Source: CAD feature listing. Evaluate the final solid. Frame: model axes, mm. A direction names the side the tool comes from. Coordinates: 2 decimals unless noted, no trailing zeros. Write each loop counter-clockwise with the first axis right and the second up, starting at its lowest first coordinate (ties: lowest second). Pieces come first, ordered by that corner, then holes. Notation, with made-up numbers: M -3,62 L 23,62 A20 ccw 23,96 Z; hole C 10,78.25 d5. An arc over 180 degrees is marked long. One line per item, written item: value. Start each with the question number.
Item 1: Set-up query: faces 1 (the cylindrical face through (-0.869, 11.059, 3.915)), 2 (the cylindrical face through (-0.33, 5.59, -2.55)). Return all of +Z, -Z, +X, -X, +Y, -Y with unobstructed straight access to the full face (end or side cutting, diameter ignored); none if empty.
Item 2: Mould query, pull axis Z, two halves, no side actions, for faces 3 (the flat face through (0, 11.22, 0)), 4 (the cylindrical face through (-2.8, 5, -0.1)), 5 (the flat face through (0, 12.07, 0)). Classes: released by +Z, released by -Z, zero draft, split by the parting line, or undercut.
Item 3: Cut plane B-B, the plane z = 0. Output: boundary loops of the cut face in (x, y), then the cut area to 3 significant figures.
Item 4: Cut plane A-A, the plane x = 0. Output: boundary loops of the cut face in (y, z).
Item 5: Ray query, L1, parallel to Z at x = 0, y = 5.75; L2, parallel to Y at x = 3, z = 0.75; L3, parallel to Z at x = 1, y = 6.5. Return the intervals inside material, ascending. Write a range as from..to.
Item 6: Cut plane C-C, the plane y = 8.25. Output: boundary loops of the cut face in (x, z), then the cut area to 3 significant figures.
Item 7: Pin query (flat end, axial travel): P1, Ø1.5, axis at y = 6, z = -3, coming from the -X side; P2, Ø3, axis at y = 5.5, z = 0.5, coming from the -X side; P3, Ø2.5, axis at x = 0.5, z = 0.5, coming from the -Y side. Return the tip coordinate at first contact, or that it passes through.
```python
from build123d import *


with BuildPart() as part:
    # Esboço1 → Revolução1 (revolve)
    with BuildSketch(Plane.XY, mode=Mode.PRIVATE) as revolu_o1_sk:
        with BuildLine():
            Line((0, 12.07), (-3.81, 12.07))
            ThreePointArc((-3.81, 12.07), (-3.951421356, 12.011421356), (-4.01, 11.87))
            Line((-4.01, 11.87), (-4.01, 10.27))
            ThreePointArc((-4.01, 10.27), (-3.951421356, 10.128578644), (-3.81, 10.07))
            Line((-3.81, 10.07), (-2.8, 10.07))
            Line((-2.8, 10.07), (-2.8, 0))
            Line((-2.8, 0), (-2.57, 0))
            Line((-2.57, 0), (-2.57, 11.02))
            ThreePointArc((-2.57, 11.02), (-2.511421356, 11.161421356), (-2.37, 11.22))
            Line((-2.37, 11.22), (0, 11.22))
            Line((0, 11.22), (0, 12.07))
        make_face()
    revolve(revolu_o1_sk.sketch.rotate(Axis((0, 0, 0), (0, 1, 0)), 180), axis=Axis((0, 0, 0), (0, 1, 0)))


solid = part.part
```
From the geometry:
1. face 1: +Y, -Y
1. face 2: -Y
2. face 3: undercut
2. face 4: split by the parting line
2. face 5: zero draft
3. outline: M -4.01,10.27 A0.2 ccw -3.81,10.07 L -2.8,10.07 L -2.8,0 L -2.57,0 L -2.57,11.02 A0.2 cw -2.37,11.22 L 2.37,11.22 A0.2 cw 2.57,11.02 L 2.57,0 L 2.8,0 L 2.8,10.07 L 3.81,10.07 A0.2 ccw 4.01,10.27 L 4.01,11.87 A0.2 ccw 3.81,12.07 L -3.81,12.07 A0.2 ccw -4.01,11.87 Z
3. area: 14.7 mm²
4. outline: M 0,-2.8 L 10.07,-2.8 L 10.07,-3.81 A0.2 ccw 10.27,-4.01 L 11.87,-4.01 A0.2 ccw 12.07,-3.81 L 12.07,3.81 A0.2 ccw 11.87,4.01 L 10.27,4.01 A0.2 ccw 10.07,3.81 L 10.07,2.8 L 0,2.8 L 0,2.57 L 11.02,2.57 A0.2 cw 11.22,2.37 L 11.22,-2.37 A0.2 cw 11.02,-2.57 L 0,-2.57 Z
5. L1: z = -2.8..-2.57, 2.57..2.8
5. L2: y = 10.07..12.07
5. L3: z = -2.62..-2.37, 2.37..2.62
6. outline: C 0,0 d5.6; hole C 0,0 d5.14
6. area: 3.88 mm²
7. P1: stops at x = -1.67
7. P2: stops at x = -2.8
7. P3: stops at y = 11.22
